from build123d import *

# Parameters (mm, degrees)
F0_R           = 12.5
F1_DEPTH       = 50
F2_R           = 10
F3_DEPTH       = 10
F4_R           = 5
F5_DEPTH       = 12
F6_W           = 3
F6_H           = 11.5
F7_DEPTH       = 12.501
F7_DEPTH_BACK  = 12.501
F8_R           = 1
F9_DEPTH       = 14.001
F9_DEPTH_BACK  = 11.001
F11_DEPTH      = 4
F12_R          = 6.75
F13_DEPTH      = 1
F13_DEPTH_BACK = 1


with BuildPart() as f1:
    # F0 (on Top) → F1 (new body)
    with BuildSketch(Plane.XY):
        Circle(F0_R)
    extrude(amount=-F1_DEPTH)

    # F2 (on Top) → F3 (join)
    with BuildSketch(Plane.XY):
        Circle(F2_R)
    extrude(amount=F3_DEPTH)

    # F4 (on face) → F5 (join)
    with BuildSketch(Plane.XY.offset(10)):
        Circle(F4_R)
    extrude(amount=F5_DEPTH)

    # F6 (on Front) → F7 (cut, two sides)
    with BuildSketch(Plane.XZ) as f7_sk:
        with Locations((0, 16.25)):
            Rectangle(F6_W, F6_H)
    extrude(amount=-F7_DEPTH, mode=Mode.SUBTRACT)
    extrude(f7_sk.sketch, amount=F7_DEPTH_BACK, mode=Mode.SUBTRACT)

    # F8 (on face) → F9 (cut, two sides)
    with BuildSketch(Plane.YZ.offset(-1.5)) as f9_sk:
        with Locations((0, 17.2303039929)):
            Circle(F8_R)
    extrude(amount=F9_DEPTH, mode=Mode.SUBTRACT)
    extrude(f9_sk.sketch, amount=-F9_DEPTH_BACK, mode=Mode.SUBTRACT)

    # F10 (on face) → F11 (join)
    with BuildSketch(Plane.XY.offset(10)):
        Polygon((6.25, -10.8253175473), (12.5, 0), (6.25, 10.8253175473), (-6.25, 10.8253175473), (-12.5, 0), (-6.25, -10.8253175473), align=None)
    extrude(amount=-F11_DEPTH)

    # F12 (on Right) → F13 (join, two sides)
    with BuildSketch(Plane.YZ) as f13_sk:
        with Locations((0, 17.2303039929)):
            Circle(F12_R)
    extrude(amount=F13_DEPTH)
    extrude(f13_sk.sketch, amount=-F13_DEPTH_BACK)


solid = f1.part
Read the model definition and answer for the solid it produces. Units are mm, in the model's axes. A direction names the side the tool comes from. Give positions to 0.01 mm unless a question says otherwise; leave off trailing zeros. Write each loop counter-clockwise with the first axis right and the second up, starting at its lowest first coordinate (ties: lowest second). Pieces come first, ordered by that corner, then holes. Notation, with made-up numbers: (28, 89) -> (50, 89) arc R24 ccw to (50, 101) -> close; hole circle Ø4 at (10.5, 61). An arc over 180 degrees is marked (long way). Answer as a JSON object with one key per item and string values. Group by question number.
1) Consider L1, parallel to Z at x = 3.45, y = 0; L2, parallel to Z at x = -5, y = 9.25; L3, parallel to X at y = -2.75, z = 17.5. Determine where each line is inside the solid, lowest interval first. Write a range as from..to.
2) A tool of negligible diameter and unlimited length cuts with its end or side. For faces 1 (the cylindrical face through (0.014, 0.29, 23.974)), 2 (the flat face through (1, 0, 17)), 3 (the flat face through (-9.33, 5.49, 8.03)), 4 (the flat face through (0, -10.825, 8)), 5 (the flat face through (9.33, -5.49, 8.03)), from which of +Z, -Z, +X, -X, +Y, -Y can it reach the whole face along a straight path? Write none if from no direction.
3) Find section D-D (x = 0). Write down the section's boundary in (y, z), and give its area (3 significant figures).
4) Find section C-C (z = -30). Write down the section's boundary in (x, y).
5) Each of these flat-tipped pins is pushed along its axis until it touches: P1, Ø3, axis at x = 1.5, z = 8, coming from the -Y side; P2, Ø1, axis at x = 8, y = 6.5, coming from the +Z side; P3, Ø3, axis at y = 4, z = -36.5, coming from the +X side. Where does it stop, or does it pass through?
6) Find section B-B (x = 7.75). Write down the section's boundary in (y, z), and give its area (3 significant figures).
7) The mould has two halves that part along X. Classify faces 6 (the flat face through (1.5, 0, 16)), 7 (the cylindrical face through (-2.17, -9.76, 2.96)), 8 (the flat face through (10.13, 0.85, 6)): +X half, -X half, draft (parallel to the pull), parting line (faces both ways), or undercut.
8) Find section A-A (y = -8.75). Write down the section's boundary in (x, z).
Values follow:
{
 "1": {"L1": "z = -50..16.23, 18.23..22", "L2": "z = -50..0, 6..10", "L3": "x = -4.18..-1.5, -1..1, 1.5..4.18"},
 "2": {"face 1": "none", "face 2": "+Z, +Y, -Y", "face 3": "+Z, -X, +Y", "face 4": "+Z, +X, -X, -Y", "face 5": "+Z, +X, -Y"},
 "3": {"outline": "(-12.5, -50) -> (12.5, -50) -> (12.5, 0) -> (10, 0) -> (10, 6) -> (10.83, 6) -> (10.83, 10) -> (5, 10) -> (5, 10.5) -> (0.52, 10.5) arc R6.75 ccw (long way) to (-0.52, 10.5) -> (-5, 10.5) -> (-5, 10) -> (-10.83, 10) -> (-10.83, 6) -> (-10, 6) -> (-10, 0) -> (-12.5, 0) -> close", "area": "1,600 mm2"},
 "4": {"outline": "circle Ø25 at (0, 0)"},
 "5": {"P1": "stops at y = -10.83", "P2": "stops at z = 10", "P3": "stops at x = 12.25"},
 "6": {"outline": "(-9.81, -50) -> (9.81, -50) -> (9.81, 0) -> (6.32, 0) -> (6.32, 6) -> (8.23, 6) -> (8.23, 10) -> (-8.23, 10) -> (-8.23, 6) -> (-6.32, 6) -> (-6.32, 0) -> (-9.81, 0) -> close", "area": "1,120 mm2"},
 "7": {"face 6": "undercut", "face 7": "parting line", "face 8": "draft"},
 "8": {"outline": "(-8.93, -50) -> (8.93, -50) -> (8.93, 0) -> (4.84, 0) -> (4.84, 6) -> (7.45, 6) -> (7.45, 10) -> (-7.45, 10) -> (-7.45, 6) -> (-4.84, 6) -> (-4.84, 0) -> (-8.93, 0) -> close"}
}
